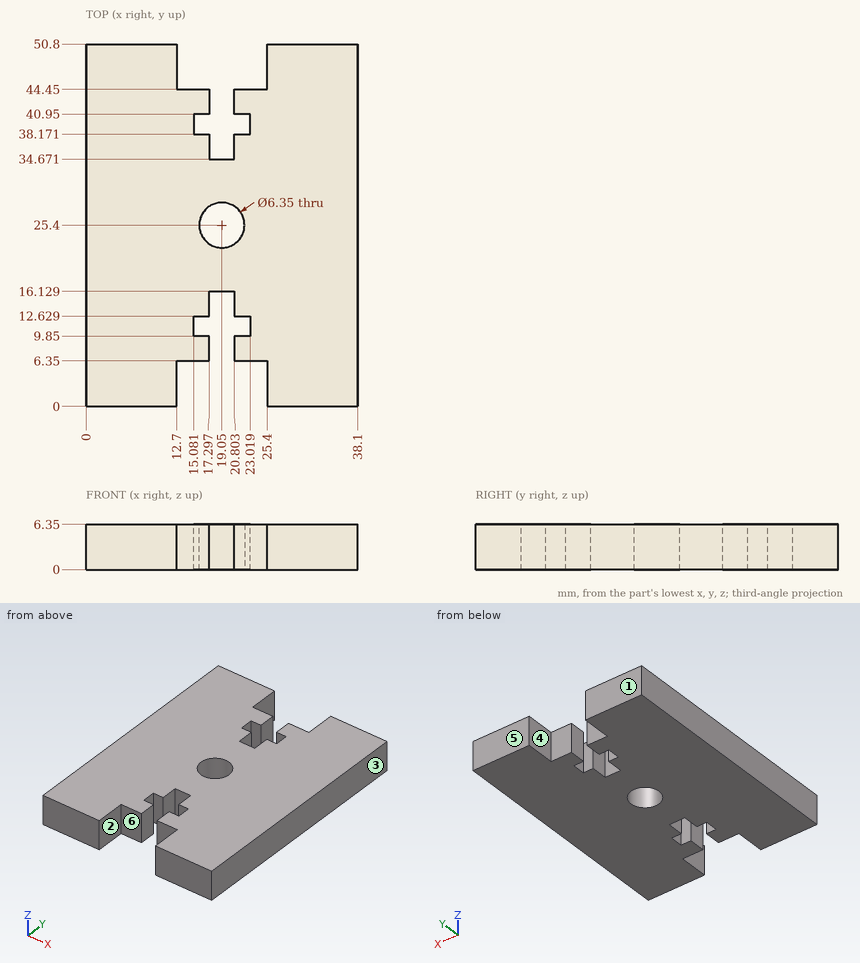
Geometry check sheet. Reference: drawing and pictorial views, mm from the part's lowest x, y, z. A direction names the side the tool comes from. Round coordinates to 2 decimals unless told otherwise and drop trailing zeros.
1. Draft check along X on the marked faces 1, 2 and 3. Enter one of: +X half, -X half, draft (parallel to the pull), parting line (faces both ways), or undercut.
2. Scan lines: L1, parallel to X at y = 11, z = 1.5; L2, parallel to X at y = 7, z = 4; L3, parallel to Y at x = 19.05, z = 2.75 (1 decimal). Record each from-to range of solid material in increasing order.
3. Gauge pin test, flat ends, axial feed: P1, Ø1.1, axis at x = 22, z = 2.5, coming from the +Y side; P2, Ø2.5, axis at x = 22.5, z = 2, coming from the -Y side; P3, Ø5, axis at x = 19.05, y = 25.4, coming from the +Z side. Record the tip position at first contact, or that the pin passes through.
4. Access from +Z, -Z, +X, -X, +Y, -Y to the whole of each face (thin tool, end or side, straight path). Record for the marked faces 4, 5 and 6.
Answer:
1. face 1: draft
1. face 2: undercut
1. face 3: +X half
2. L1: x = 0 to 15.08, 23.02 to 38.1
2. L2: x = 0 to 17.3, 20.8 to 38.1
2. L3: y = 16.1 to 22.2, 28.6 to 34.7
3. P1: stops at y = 44.45
3. P2: stops at y = 6.35
3. P3: passes through
4. face 4: +Z, -Z, +Y
4. face 5: +Z, -Z, +X, -X, +Y
4. face 6: +Z, -Z, -Y
